Can you work these out from the drawing? Everything is in mm from the part's minimum corner. Round coordinates to 2 decimals unless told otherwise and drop trailing zeros. Loops run counter-clockwise (first coordinate to the right, second up) from the corner with the lowest first, then second, coordinate; pieces in that order, holes last. Notation, with made-up numbers: M -3,88 L 56,88 A36 cw 56,122 Z; hole C 62.25,80.25 d5. An arc over 180 degrees is marked long. One line per question, with ' | ' between items. Start each with the question number.
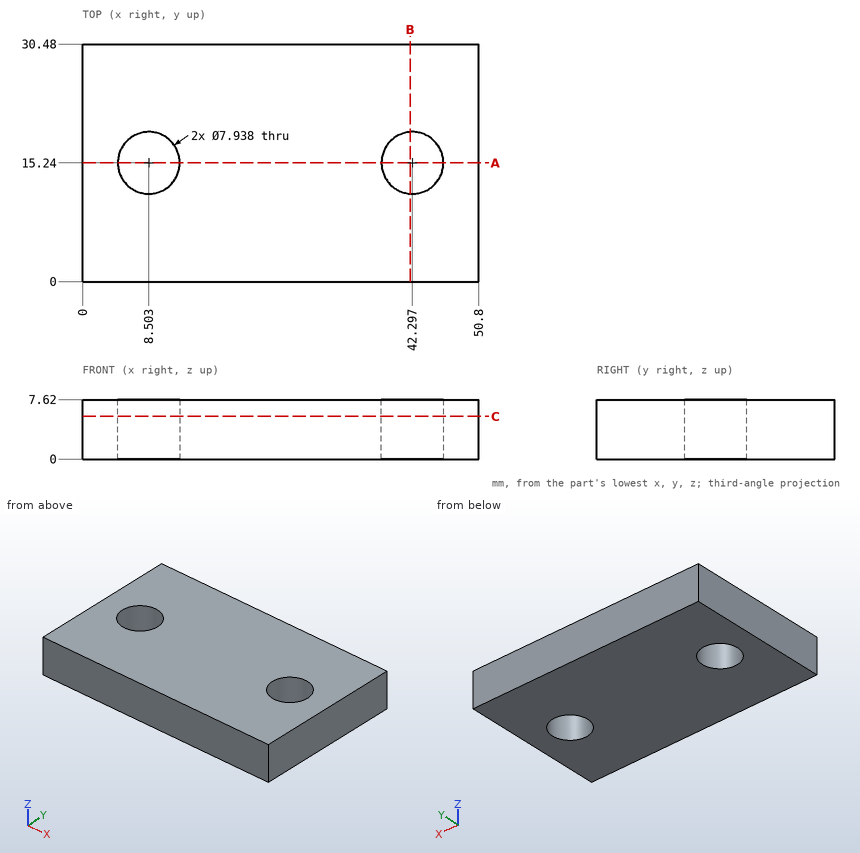
1) I'm going to push a flat-ended pin straight in: pin 1 Ø7 at (x, y) = (8.5, 15.24) entering from +Z. Where does the tip first touch, or does it pass through?
2) Imagine slicing it at B-B (x = 42). Write out the boundary of the cut face in (y, z), then the cut area to 3 significant figures.
3) Please list where these lines run through material, in increasing order: L1, parallel to X at y = 18.5, z = 1.75 (1 decimal); L2, parallel to X at y = 13, z = 7 (1 decimal); L3, parallel to Y at x = 11.5, z = 6. Write a range as from..to.
4) Imagine slicing it at C-C (z = 5.5). Write out the boundary of the cut face in (x, y), then the cut area to 3 significant figures.
5) Imagine slicing it at A-A (y = 15.24). Write out the boundary of the cut face in (x, z), then the cut area to 3 significant figures.
Results are:
1) pin 1: through
2) outline: M 0,0 L 11.28,0 L 11.28,7.62 L 0,7.62 Z; M 19.2,0 L 30.48,0 L 30.48,7.62 L 19.2,7.62 Z | area: 172 mm²
3) L1: 0..6.2, 10.8..40, 44.6..50.8 | L2: 0..5.2, 11.8..39, 45.6..50.8 | L3: 0..12.64, 17.84..30.48
4) outline: M 0,0 L 50.8,0 L 50.8,30.48 L 0,30.48 Z; hole C 8.5,15.24 d7.94; hole C 42.3,15.24 d7.94 | area: 1,450 mm²
5) outline: M 0,0 L 4.53,0 L 4.53,7.62 L 0,7.62 Z; M 12.47,0 L 38.33,0 L 38.33,7.62 L 12.47,7.62 Z; M 46.27,0 L 50.8,0 L 50.8,7.62 L 46.27,7.62 Z | area: 266 mm²
